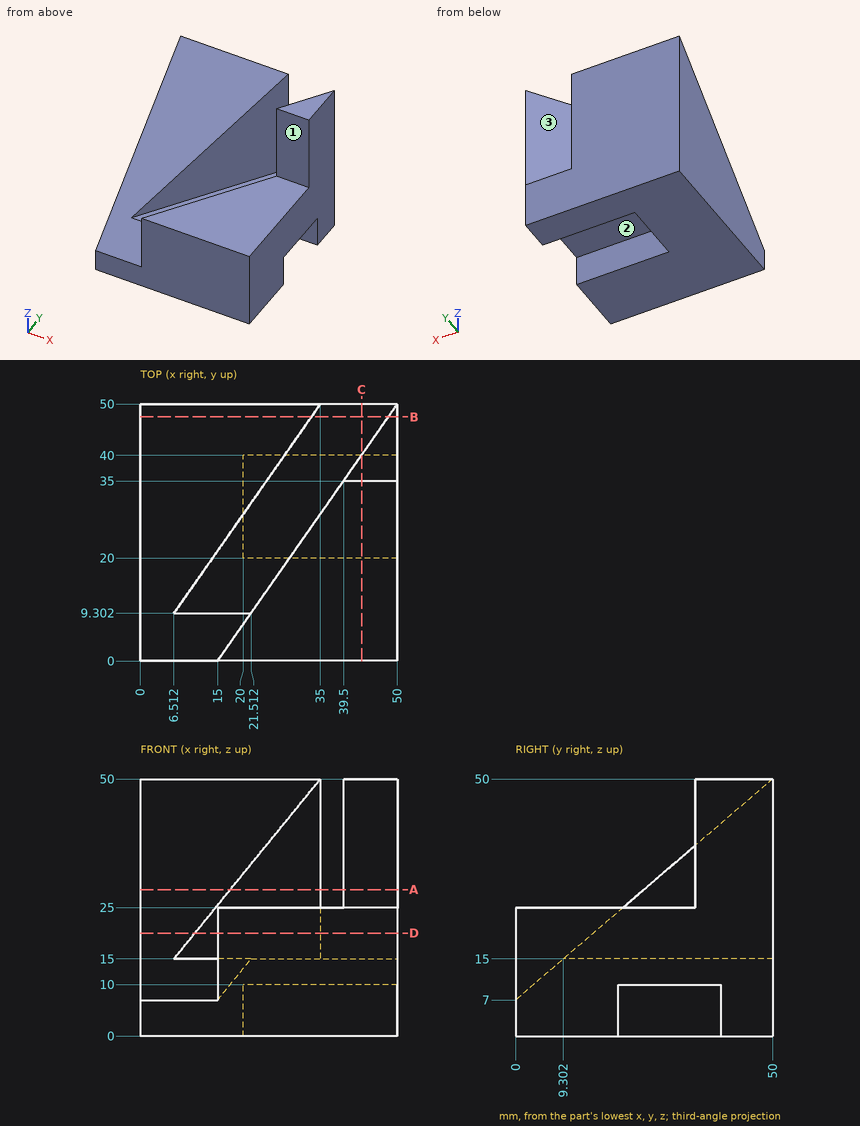
Drawing for the job (mm, zero at the part's lowest x, y, z). A direction names the side the tool comes from. Round coordinates to 2 decimals unless told otherwise and drop trailing zeros. Write each loop counter-clockwise with the first axis right and the second up, starting at its lowest first coordinate (ties: lowest second). Pieces come first, ordered by that corner, then holes. Notation, with made-up numbers: (-26, 42) - (33, 42) arc R19 ccw to (33, 69) - close; hole circle Ø6 at (77, -25). An arc over 180 degrees is marked (long way). Return JSON: item names as keys, results as strings. Group by question number.
Item 1: Band-saw the part on D-D on z = 20. List the corners of the cut face in (x, y).
Item 2: 3-axis set-ups, long thin cutter, end or side, ignore diameter. For the marked faces 1, 2 and 3: which of +Z, -Z, +X, -X, +Y, -Y reach the whole face in a straight line?
Item 3: Probe probe 1 along Z at (x, y) = (22.5, 16.5); probe 2 along Z at (x, y) = (48, 24.5); probe 3 along X at (y, z) = (41.5, 37). List the from-to ranges inside material, lowest first.
Item 4: Band-saw the part on A-A on z = 28.5. List the corners of the cut face in (x, y), plus the area to 3 significant figures.
Item 5: Flat gauge pins, fed straight in: pin 1 Ø20.5 at (x, y) = (27, 28) entering from +Z; pin 2 Ø8 at (x, z) = (23, 40.5) entering from -Y; pin 3 Ø11.5 at (x, z) = (43, 40.5) entering from -Y; pin 4 Ø1 at (y, z) = (10, 27) entering from -X. Where does each tip first touch, or does it go through?
Item 6: Band-saw the part on B-B on y = 47.5. List the corners of the cut face in (x, z).
Item 7: Band-saw the part on C-C on x = 43. List the corners of the cut face in (y, z), plus the area to 4 significant figures.
Resolved:
{
 "1": {"outline": "(0, 15.12) - (10.58, 15.12) - (35, 50) - (0, 50) - close; (15, 0) - (50, 0) - (50, 50) - close"},
 "2": {"face 1": "+Z, +X, -Y", "face 2": "-Z, +X", "face 3": "+Z"},
 "3": {"probe 1": "z = 0 to 15", "probe 2": "z = 10 to 25", "probe 3": "x = 0 to 29.05, 44.05 to 50"},
 "4": {"outline": "(0, 25) - (17.5, 25) - (35, 50) - (0, 50) - close; (39.5, 35) - (50, 35) - (50, 50) - close", "area": "735 mm²"},
 "5": {"pin 1": "stops at z = 39.89", "pin 2": "stops at y = 34.3", "pin 3": "stops at y = 35", "pin 4": "passes through"},
 "6": {"outline": "(0, 0) - (50, 0) - (50, 50) - (48.25, 50) - (48.25, 15) - (33.25, 15) - (33.25, 47.85) - (0, 47.85) - close"},
 "7": {"outline": "(0, 0) - (20, 0) - (20, 10) - (40, 10) - (40, 0) - (50, 0) - (50, 15) - (40, 15) - (40, 50) - (35, 50) - (35, 25) - (0, 25) - close", "area": "1,075 mm²"}
}
